Can you work these out from the model? Positions are in its coordinate system, mm. Face numbers are marked on the shaded views. Coordinates: 2 decimals unless noted, no trailing zeros. Loops run counter-clockwise (first coordinate to the right, second up) from the corner with the lowest first, then second, coordinate; pieces in that order, holes last. Notation, with made-up numbers: (-1, 35.25) -> (36, 35.25) arc R24 ccw to (36, 56.25) -> close; hole circle Ø11 at (23, 7). An arc over 180 degrees is marked (long way). Put each result on its own line as item: value. Start each with the question number.
Item 1: Please list where these lines run through material, in increasing order: L1, parallel to X at y = 6, z = 54; L2, parallel to X at y = 54, z = 53; L3, parallel to X at y = 64, z = 23. Write a range as from..to.
Item 2: If we section it at A-A on x = 0: Please give me the cut outline in (y, z), plus the area to 3 significant figures.
Item 3: If we section it at D-D on y = 45.5: Please give me the cut outline in (x, z), plus the area to 3 significant figures.
Item 4: If we section it at B-B on y = 54.61: Please give me the cut outline in (x, z), plus the area to 3 significant figures.
Item 5: If we section it at C-C on z = 0: Please give me the cut outline in (x, y), plus the area to 3 significant figures.
Item 6: We'd pull the mould along Z, two halves only. Please class the marked faces 1, 2, 3 and 4: pulls with the +Z half, pulls with the -Z half, needs draft (parallel to the pull), parting line crosses it, or undercut.
Item 7: Will these pins go through, and if not, where does the flat tip stop? P1, Ø1, axis at y = 19.5, z = 8, coming from the -X side; P2, Ø3, axis at y = 58, z = 9, coming from the +X side; P3, Ø6.5, axis at x = 58.42, y = 69.85, coming from the +Z side; P4, Ø10, axis at x = -16, y = 49, coming from the -Z side.
```python
from build123d import *

# Parameters (mm, degrees)
SKETCH1_R           = 57.15
SKETCH1_R_2         = 50.8
BOSS_EXTRUDE1_DEPTH = 76.2
FILLET3_R           = 10
SKETCH2_R           = 2.413
CUT_EXTRUDE1_DEPTH  = 147.601134034


with BuildPart() as part:
    # Sketch1 → Boss-Extrude1 (new body)
    # profile 1 of 4: a face of its own
    with BuildSketch(Plane(origin=(0, 0, 0), x_dir=(1, 0, 0), z_dir=(0, 1, 0))):
        Circle(SKETCH1_R)
        with Locations(Location((0, 0, 0), (0, 0, 90))):
            Circle(SKETCH1_R_2, mode=Mode.SUBTRACT)
    # profile 2 of 4: a face of its own
    with BuildSketch(Plane(origin=(0, 0, 0), x_dir=(1, 0, 0), z_dir=(0, 1, 0))):
        with BuildLine():
            Line((-63.5, -57.15), (1.05e-07, -57.15))
            ThreePointArc((1.05e-07, -57.15), (-13.470384131, -55.539816811), (-26.181720723, -50.8))
            Line((-26.181720723, -50.8), (-63.5, -50.8))
            Line((-63.5, -50.8), (-63.5, -57.15))
        make_face()
    # profile 3 of 4: a face of its own
    with BuildSketch(Plane(origin=(0, 0, 0), x_dir=(1, 0, 0), z_dir=(0, 1, 0))):
        with BuildLine():
            ThreePointArc((-26.181720723, -50.8), (-13.470384131, -55.539816811), (1.05e-07, -57.15))
            ThreePointArc((1.05e-07, -57.15), (13.470384232, -55.539816786), (26.181720723, -50.8))
            Line((26.181720723, -50.8), (9.7e-08, -50.8))
            Line((9.7e-08, -50.8), (-26.181720723, -50.8))
        make_face()
    # profile 4 of 4: a face of its own
    with BuildSketch(Plane(origin=(0, 0, 0), x_dir=(1, 0, 0), z_dir=(0, 1, 0))):
        with BuildLine():
            Line((1.05e-07, -57.15), (63.5, -57.15))
            Line((63.5, -57.15), (63.5, -50.8))
            Line((63.5, -50.8), (26.181720723, -50.8))
            ThreePointArc((26.181720723, -50.8), (13.470384232, -55.539816786), (1.05e-07, -57.15))
        make_face()
    extrude(amount=BOSS_EXTRUDE1_DEPTH)

    # Fillet3
    fillet3_edges = [part.edges().sort_by_distance(p)[0] for p in [
        (26.181720723, 38.1, 50.8),
        (-26.181720723, 38.1, 50.8),
    ]]
    fillet(fillet3_edges, radius=FILLET3_R)

    # Sketch2 → Cut-Extrude1 (cut, through all)
    with BuildSketch(Plane(origin=(0, 0, 50.8), x_dir=(-1, 0, 0), z_dir=(0, 0, -1))):
        with Locations((58.416845051, 6.35)):
            Circle(SKETCH2_R)
        with Locations((58.416845051, 21.59)):
            Circle(SKETCH2_R)
        with Locations((58.416845051, 69.85)):
            Circle(SKETCH2_R)
        with Locations((58.416845051, 54.61)):
            Circle(SKETCH2_R)
        with Locations((-58.416845051, 6.35)):
            Circle(SKETCH2_R)
        with Locations((-58.416845051, 21.59)):
            Circle(SKETCH2_R)
        with Locations((-58.416845051, 69.85)):
            Circle(SKETCH2_R)
        with Locations((-58.416845051, 54.61)):
            Circle(SKETCH2_R)
    extrude(amount=-CUT_EXTRUDE1_DEPTH, mode=Mode.SUBTRACT)


solid = part.part
```
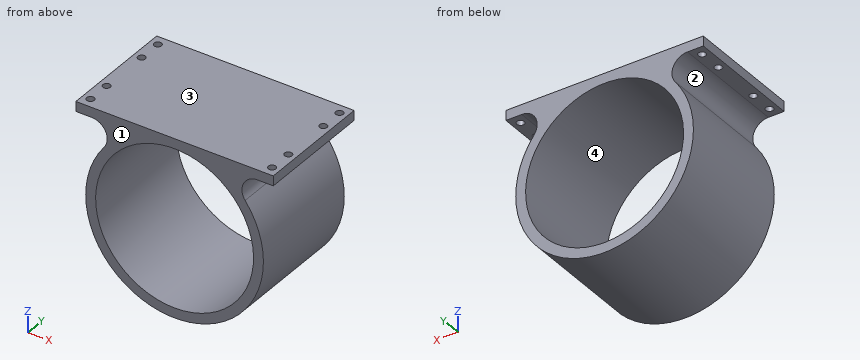
Solutions:
1. L1: -63.5..-60.8, -56.03..56.03, 60.8..63.5
1. L2: -63.5..-60.75, -56.08..56.08, 60.75..63.5
1. L3: -52.32..-45.3, 45.3..52.32
2. outline: (0, -57.15) -> (76.2, -57.15) -> (76.2, -50.8) -> (0, -50.8) -> close; (0, 50.8) -> (76.2, 50.8) -> (76.2, 57.15) -> (0, 57.15) -> close
2. area: 968 mm^2
3. outline: (-63.5, 50.8) -> (-53.33, 50.8) arc R10 cw to (-45.39, 34.72) arc R57.15 ccw (long way) to (45.39, 34.72) arc R10 cw to (53.33, 50.8) -> (63.5, 50.8) -> (63.5, 57.15) -> (-63.5, 57.15) -> close; hole circle Ø101.6 at (0, 0)
3. area: 2,980 mm^2
4. outline: (-63.5, 50.8) -> (-60.83, 50.8) -> (-60.83, 57.15) -> (-63.5, 57.15) -> close; (-56, 50.8) -> (-53.33, 50.8) arc R10 cw to (-45.39, 34.72) arc R57.15 ccw (long way) to (45.39, 34.72) arc R10 cw to (53.33, 50.8) -> (56, 50.8) -> (56, 57.15) -> (-56, 57.15) -> close; (60.83, 50.8) -> (63.5, 50.8) -> (63.5, 57.15) -> (60.83, 57.15) -> close; hole circle Ø101.6 at (0, 0)
4. area: 2,920 mm^2
5. outline: (-57.15, 0) -> (-50.8, 0) -> (-50.8, 76.2) -> (-57.15, 76.2) -> close; (50.8, 0) -> (57.15, 0) -> (57.15, 76.2) -> (50.8, 76.2) -> close
5. area: 968 mm^2
6. face 1: needs draft
6. face 2: undercut
6. face 3: pulls with the +Z half
6. face 4: undercut
7. P1: x = -56.66
7. P2: x = 56.66
7. P3: z = 57.15
7. P4: z = -56.08
